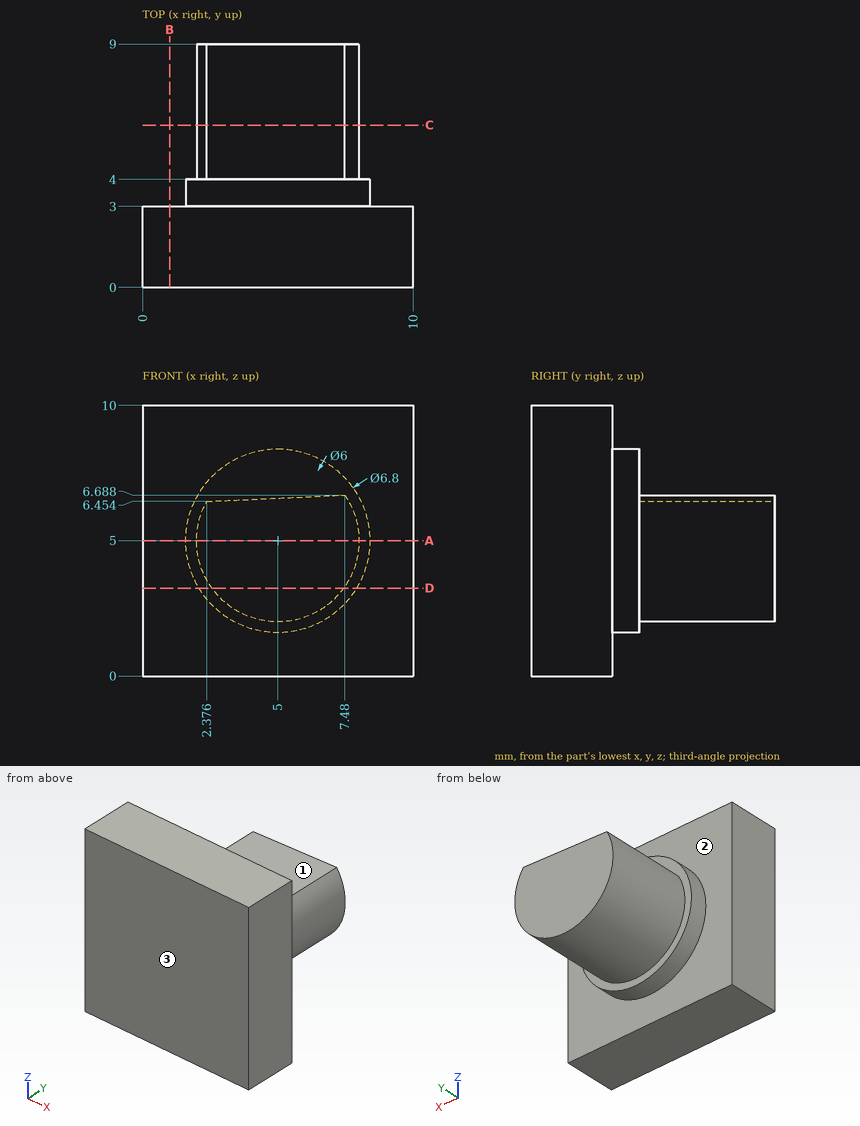
Geometry check sheet. Reference: drawing and pictorial views, mm from the part's lowest x, y, z. A direction names the side the tool comes from. Give positions to 0.01 mm unless a question says otherwise; leave off trailing zeros. Loops run counter-clockwise (first coordinate to the right, second up) from the corner with the lowest first, then second, coordinate; pieces in that order, holes last.
1. Set-up check for the marked faces 1, 2 and 3: record each of +Z, -Z, +X, -X, +Y, -Y from which the full face is reachable in a straight line by a thin tool's end or side.
2. Section check C-C, the plane y = 6. Enter the section's corners in (x, z).
3. Thickness scan on line 1 (Y direction, x = 3.75, z = 7.75); line 2 (Y direction, x = 6.5, z = 9); line 3 (X direction, y = 3.75, z = 5). Record the ranges inside material, lowest first.
4. Section check D-D, the plane z = 3.25. Enter the section's corners in (x, y) (1 decimal), then the cut area to 3 significant figures.
5. Section check A-A, the plane z = 5. Enter the section's corners in (x, y).
6. Section check B-B, the plane x = 1. Enter the section's corners in (y, z).
7. Go/stop test with flat-tipped pins: pin 1 Ø4 at (y, z) = (3.5, 7.5) entering from +X; pin 2 Ø2 at (x, y) = (2.5, 6.5) entering from -Z; pin 3 Ø1 at (x, y) = (3.5, 5) entering from -Z. Record where each tip stops, or that it passes through.
Geometry says:
1. face 1: +Z, -X, +Y
1. face 2: +Y
1. face 3: +Z, -Z, +X, -X, -Y
2. outline: (2.38, 6.45) arc R3 ccw (long way) to (7.48, 6.69) - close
3. line 1: y = 0 to 4
3. line 2: y = 0 to 3
3. line 3: x = 1.6 to 8.4
4. outline: (0, 0) - (10, 0) - (10, 3) - (7.9, 3) - (7.9, 4) - (7.4, 4) - (7.4, 9) - (2.6, 9) - (2.6, 4) - (2.1, 4) - (2.1, 3) - (0, 3) - close
4. area: 60.2 mm2
5. outline: (0, 0) - (10, 0) - (10, 3) - (8.4, 3) - (8.4, 4) - (8, 4) - (8, 9) - (2, 9) - (2, 4) - (1.6, 4) - (1.6, 3) - (0, 3) - close
6. outline: (0, 0) - (3, 0) - (3, 10) - (0, 10) - close
7. pin 1: stops at x = 10
7. pin 2: stops at z = 2.4
7. pin 3: stops at z = 2.17
